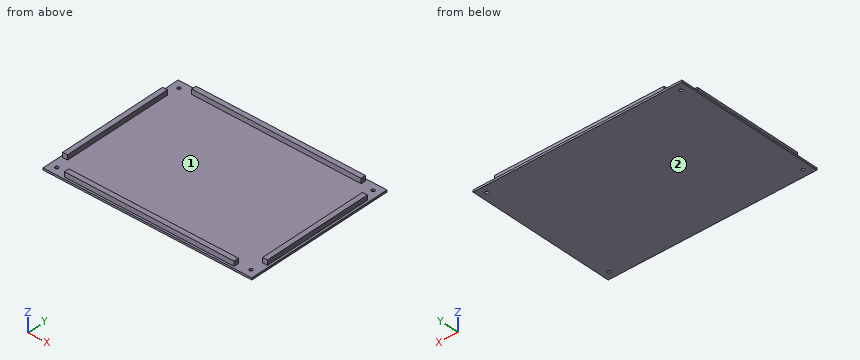
```python
from build123d import *

# Parameters (mm, degrees)
F0_W     = 214
F0_H     = 154
F1_DEPTH = 2
F2_W     = 5
F2_H     = 113.8
F2_W_2   = 173.8
F2_H_2   = 5
F3_DEPTH = 5
F5_D     = 3.4
F5_DEPTH = 5
F5_TIP   = 1.0214630523


# Not quite as in the source:
# - a feature names something its author has since deleted; it is built from what else it names


with BuildPart() as f1:
    # F0 (on Top) → F1 (new body)
    with BuildSketch(Plane.XY):
        Rectangle(F0_W, F0_H)
    extrude(amount=F1_DEPTH)

    # F2 (on face) → F3 (join)
    with BuildSketch(Plane.XY.offset(2)):
        with Locations((-102.4, 0)):
            Rectangle(F2_W, F2_H)
        with Locations((0, 72.4)):
            Rectangle(F2_W_2, F2_H_2)
        with Locations((102.4, 0)):
            Rectangle(F2_W, F2_H)
        with Locations((0, -72.4)):
            Rectangle(F2_W_2, F2_H_2)
    extrude(amount=F3_DEPTH)

    # F5
    with Locations(Plane(origin=(0, 0, 0), x_dir=(1, 0, 0), z_dir=(0, 0, -1))):
        with Locations((-99.5, -69.5), (-99.5, 69.5), (99.5, 69.5), (99.5, -69.5)):
            Hole(F5_D / 2, depth=F5_DEPTH)
            with Locations((0, 0, -(F5_DEPTH + F5_TIP / 2))):  # 118° drill point
                Cone(0, F5_D / 2, F5_TIP, mode=Mode.SUBTRACT)


solid = f1.part
```
Geometry check sheet. Reference: the model listing, model coordinates, mm. Face numbers are marked on the shaded views. Give positions to 0.01 mm unless a question says otherwise; leave off trailing zeros. Write each loop counter-clockwise with the first axis right and the second up, starting at its lowest first coordinate (ties: lowest second). Pieces come first, ordered by that corner, then holes. Notation, with made-up numbers: (2.5, -23) - (49.5, -23) arc R19 ccw to (49.5, 2) - close; hole circle Ø1 at (50, 23.5). An arc over 180 degrees is marked (long way). Use a Markdown table: item, result.
Q1. Section check D-D, the plane y = -63.5. Enter the section's corners in (x, z), then the cut area to 3 significant figures.
Computed:
| item | result |
|---|---|
| outline | (-107, 0) - (107, 0) - (107, 2) - (-107, 2) - close |
| area | 428 mm² |
Q2. Go/stop test with flat-tipped pins: P1, Ø4, axis at y = 72.5, z = 4.5, coming from the -X side; P2, Ø2, axis at x = -80, z = 4, coming from the +Y side; P3, Ø5.5, axis at x = 99.5, y = -69.5, coming from the -Z side; P4, Ø2, axis at y = -27, z = 3.5, coming from the -X side. Record where each tip stops, or that it passes through.
Computed:
| item | result |
|---|---|
| P1 | stops at x = -86.9 |
| P2 | stops at y = 74.9 |
| P3 | stops at z = 0 |
| P4 | stops at x = -104.9 |
Q3. Draft check along X on the marked faces 1 and 2. Enter one of: pulls with the +X half, pulls with the -X half, needs draft (parallel to the pull), parting line crosses it, or undercut.
Computed:
| item | result |
|---|---|
| face 1 | undercut |
| face 2 | needs draft |
Q4. Section check C-C, the plane y = -11. Enter the section's corners in (x, z), then the cut area to 3 significant figures.
Computed:
| item | result |
|---|---|
| outline | (-107, 0) - (107, 0) - (107, 2) - (104.9, 2) - (104.9, 7) - (99.9, 7) - (99.9, 2) - (-99.9, 2) - (-99.9, 7) - (-104.9, 7) - (-104.9, 2) - (-107, 2) - close |
| area | 478 mm² |
Q5. Section check A-A, the plane z = 5.75. Enter the section's corners in (x, y), then the cut area to 3 significant figures.
Computed:
| item | result |
|---|---|
| outline | (-104.9, -56.9) - (-99.9, -56.9) - (-99.9, 56.9) - (-104.9, 56.9) - close; (-86.9, -74.9) - (86.9, -74.9) - (86.9, -69.9) - (-86.9, -69.9) - close; (-86.9, 69.9) - (86.9, 69.9) - (86.9, 74.9) - (-86.9, 74.9) - close; (99.9, -56.9) - (104.9, -56.9) - (104.9, 56.9) - (99.9, 56.9) - close |
| area | 2,880 mm² |
Q6. Thickness scan on L1, parallel to Y at x = 99.5, z = 1.05; L2, parallel to Y at x = 49, z = 5.25; L3, parallel to X at y = -69.5, z = 0.95. Record the ranges inside material, lowest first. Write a range as [from, to].
Computed:
| item | result |
|---|---|
| L1 | y = [-77, -71.2], [-67.8, 67.8], [71.2, 77] |
| L2 | y = [-74.9, -69.9], [69.9, 74.9] |
| L3 | x = [-107, -101.2], [-97.8, 97.8], [101.2, 107] |
Q7. Section check B-B, the plane x = -4. Enter the section's corners in (y, z).
Computed:
| item | result |
|---|---|
| outline | (-77, 0) - (77, 0) - (77, 2) - (74.9, 2) - (74.9, 7) - (69.9, 7) - (69.9, 2) - (-69.9, 2) - (-69.9, 7) - (-74.9, 7) - (-74.9, 2) - (-77, 2) - close |
